Answer from the drawing. Dimensions are ordinates in mm from the lowest x, y and z of the part. Give positions to 0.01 mm unless a question says otherwise; leave off trailing zeros. Loops run counter-clockwise (first coordinate to the right, second up) from the corner with the lowest first, then second, coordinate; pieces in that order, holes last.
(1) Find section A-A, the plane y = 24.5. Write down the section's boundary in (x, z), then the cut area to 3 significant figures.
(2) This flat-tipped pin is pushed along its axis until it touches: P1, Ø10, axis at x = 36.5, y = 19, coming from the -Z side. Where does it stop, or does it pass through?
(3) Straight lines are drawn through the part: probe 1 along Y at (x, z) = (24.5, 3.2); probe 2 along X at (y, z) = (8, 1.45); probe 3 along X at (y, z) = (10, 0.6). For each, find the intervals that lie inside material, in ascending order.
(4) Determine the mould class of the marked faces 1 and 2 for opening direction X: pulls with the +X half, pulls with the -X half, needs draft (parallel to the pull), parting line crosses it, or undercut.
(5) Find section C-C, the plane z = 1.9. Write down the section's boundary in (x, y), then the cut area to 3 significant figures.
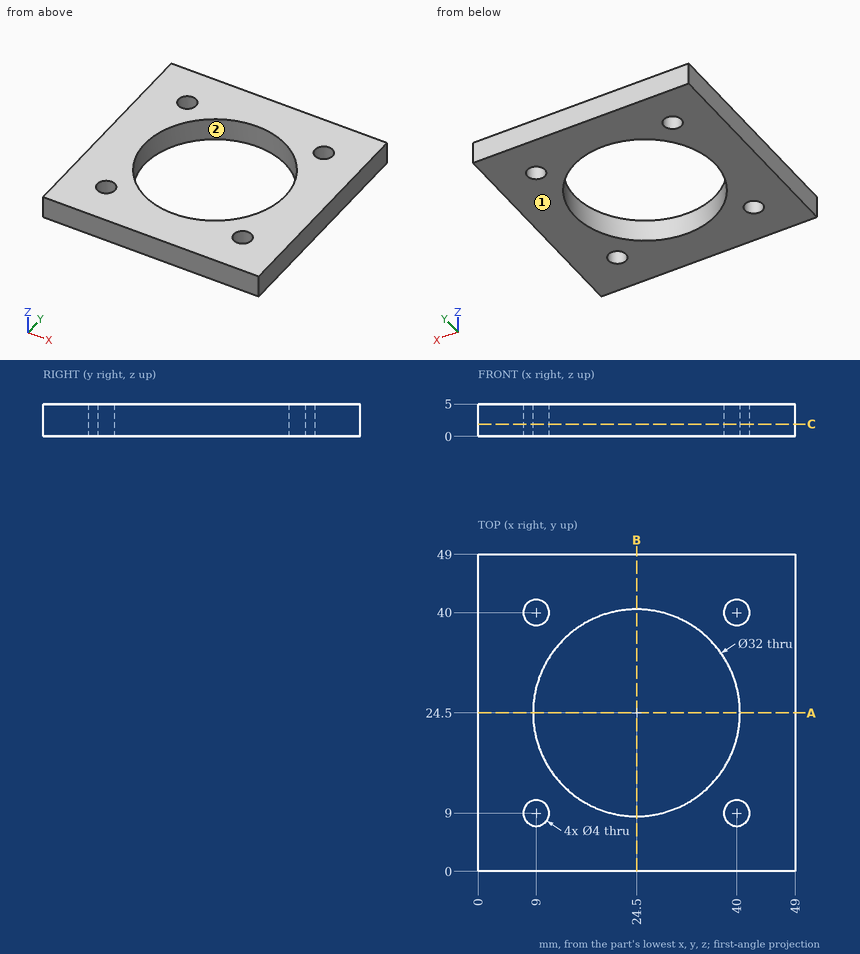
Entries:
1. outline: (0, 0) - (8.5, 0) - (8.5, 5) - (0, 5) - close; (40.5, 0) - (49, 0) - (49, 5) - (40.5, 5) - close
1. area: 85.0 mm2
2. P1: stops at z = 0
3. probe 1: y = 0 to 8.5, 40.5 to 49
3. probe 2: x = 0 to 7.27, 10.73 to 38.27, 41.73 to 49
3. probe 3: x = 0 to 7.27, 10.73 to 17.74, 31.26 to 38.27, 41.73 to 49
4. face 1: needs draft
4. face 2: undercut
5. outline: (0, 0) - (49, 0) - (49, 49) - (0, 49) - close; hole circle Ø4 at (9, 9); hole circle Ø4 at (9, 40); hole circle Ø32 at (24.5, 24.5); hole circle Ø4 at (40, 9); hole circle Ø4 at (40, 40)
5. area: 1,550 mm2
